Autodesk Fusion 360 part; units mm, degrees
sketch "Body" plane through (0, 0, 0) normal (0, 0, 1) x (1, 0, 0)
  circle A0 centre (0, 0) radius 85
  line L0 (-100, -41.4214) -> (-41.4214, -100)
  line L1 (-41.4214, -100) -> (41.4214, -100)
  line L2 (41.4214, -100) -> (100, -41.4214)
  line L3 (100, -41.4214) -> (100, 41.4214)
  line L4 (100, 41.4214) -> (41.4214, 100)
  line L5 (41.4214, 100) -> (-41.4214, 100)
  line L6 (-41.4214, 100) -> (-100, 41.4214)
  line L7 (-100, 41.4214) -> (-100, -41.4214)
  line L8 (-30.5, -100) -> (30.5, -100)
  line L9 (30.5, -100) -> (30.5, -120)
  line L10 (30.5, -120) -> (-30.5, -120)
  line L11 (-30.5, -120) -> (-30.5, -100)
  line L12 (-30.5, 100) -> (30.5, 100)
  line L13 (30.5, 100) -> (30.5, 120)
  line L14 (30.5, 120) -> (-30.5, 120)
  line L15 (-30.5, 120) -> (-30.5, 100)
  line L16 (100, 30.5) -> (120, 30.5)
  line L17 (120, 30.5) -> (120, -30.5)
  line L18 (120, -30.5) -> (100, -30.5)
  line L19 (100, -30.5) -> (100, 30.5)
  line L20 (-100, 30.5) -> (-120, 30.5)
  line L21 (-120, 30.5) -> (-120, -30.5)
  line L22 (-120, -30.5) -> (-100, -30.5)
  line L23 (-100, -30.5) -> (-100, 30.5)
  line L24 (-120, 0) -> (120, 0)
  line L25 (0, 120) -> (0, -120)
  dimension "d1" = 170
  dimension "d2" = 100
  dimension "d4" = 61
  dimension "d5" = 20
  dimension "d7" = 61
  dimension "d8" = 20
  dimension "d10" = 61
  dimension "d11" = 20
  dimension "d13" = 20
  dimension "d14" = 61
extrude "Extrude1" add sketch "Body" along normal blind 100 contours A0 L3 L4 L5 L12 L19 L24 L25 | L3 L16 L17 L19 L24 | L5 L12 L13 L14 L25
extrude "Extrude2" cut sketch "Body" along normal blind 7 contours L3 L16 L17 L19 L24 | L5 L12 L13 L14 L25
sketch "H_Circle" plane through (30.5, 0, 0) normal (1, 0, 0) x (0, 1, 0)
  line L0 (100, 7) -> (120, 7)
  line L1 (120, 7) -> (120, 100)
  line L2 (120, 100) -> (100, 100)
  line L3 (100, 100) -> (100, 7)
  line L4 (100, 100) -> (120, 100)
  line L5 (120, 100) -> (120, 7)
  line L6 (120, 7) -> (100, 7)
  line L7 (100, 7) -> (100, 100)
  line L8 (100, 100) -> (120, 100)
  line L9 (120, 100) -> (120, 80)
  line L10 (100, 80) -> (100, 100)
  line L11 (100, 7) -> (120, 7)
  line L12 (120, 7) -> (120, 27)
  line L13 (100, 27) -> (100, 7)
  circle A0 centre (110, 80) radius 6
  circle A1 centre (110, 80) radius 3
  circle A2 centre (110, 27) radius 6
  circle A3 centre (110, 27) radius 3
  dimension "d19" = 20
  dimension "d20" = 20
  dimension "d21" = 12
  dimension "d22" = 6
  dimension "d23" = 12
  dimension "d24" = 6
extrude "Extrude3" cut sketch "H_Circle" against normal blind 70 contours A1 | A3
extrude "Extrude4" cut sketch "H_Circle" against normal blind 6 contours A0 | A2
sketch "H_Hex" plane through (0, 30.5, 0) normal (0, 1, 0) x (-1, 0, 0)
  line L0 (-120, 7) -> (-100, 7)
  line L1 (-100, 7) -> (-100, 100)
  line L2 (-100, 100) -> (-120, 100)
  line L3 (-120, 100) -> (-120, 7)
  line L4 (-120, 100) -> (-100, 100)
  line L5 (-100, 100) -> (-100, 7)
  line L6 (-100, 7) -> (-120, 7)
  line L7 (-120, 7) -> (-120, 100)
  line L8 (-120, 100) -> (-100, 100)
  line L9 (-100, 100) -> (-100, 80)
  line L10 (-120, 80) -> (-120, 100)
  line L11 (-120, 7) -> (-100, 7)
  line L12 (-100, 7) -> (-100, 27)
  line L13 (-120, 27) -> (-120, 7)
  circle A0 centre (-110, 80) radius 3
  circle A1 centre (-110, 27) radius 3
  line L14 (-115.5, 76.8246) -> (-110, 73.6491)
  line L15 (-110, 73.6491) -> (-104.5, 76.8246)
  line L16 (-104.5, 76.8246) -> (-104.5, 83.1754)
  line L17 (-104.5, 83.1754) -> (-110, 86.3509)
  line L18 (-110, 86.3509) -> (-115.5, 83.1754)
  line L19 (-115.5, 83.1754) -> (-115.5, 76.8246)
  line L20 (-115.5, 23.8246) -> (-110, 20.6491)
  line L21 (-110, 20.6491) -> (-104.5, 23.8246)
  line L22 (-104.5, 23.8246) -> (-104.5, 30.1754)
  line L23 (-104.5, 30.1754) -> (-110, 33.3509)
  line L24 (-110, 33.3509) -> (-115.5, 30.1754)
  line L25 (-115.5, 30.1754) -> (-115.5, 23.8246)
  point P0 (-110, 80)
  point P1 (-110, 27)
  dimension "d30" = 20
  dimension "d31" = 20
  dimension "d32" = 6
  dimension "d33" = 6
  dimension "d34" = 5.5
  dimension "d35" = 5.5
extrude "Extrude5" cut sketch "H_Hex" against normal blind 5 contours L14 L15 L16 L17 L18 L19 | L20 L21 L22 L23 L24 L25
extrude "Extrude6" cut 2 faces at (110.2225, 30.5, 80.9749) (109.2094, 30.5, 26.0676) along direction (0, -1, 0) blind 80
Geometry check sheet. Reference: the model listing, model coordinates, mm. A direction names the side the tool comes from. Coordinates: 2 decimals unless noted, no trailing zeros. Order: outer loops, then holes, each group sorted by start corner. A loop starts at its lowest first (then second) coordinate and runs counter-clockwise, first axis right, second up. Notation, with made-up numbers: (29, 81.5) - (37, 81.5) arc R5 cw to (37, 87.5) - close; hole circle Ø3 at (55.25, 44.25). An arc over 180 degrees is marked (long way). Answer in a Markdown table with one row per item. Add a question column.
1. Section check C-C (z = 14). Enter the section's corners in (x, y), plus the area to 3 significant figures.
2. Section check B-B (y = 14.5). Enter the section's corners in (x, z).
3. Gauge pin test, flat ends, axial feed: pin 1 Ø10 at (x, y) = (10, 113) entering from -Z; pin 2 Ø6 at (x, z) = (25, 23) entering from -Y; pin 3 Ø3.5 at (y, z) = (107.5, 77.5) entering from +X; pin 4 Ø6 at (x, y) = (36.5, 71.5) entering from +Z. Record the tip position at first contact, or that the pin passes through.
4. Draft check along Y on faces 1 (the face through (27.54, 105.58, 84.06)), 2 (the face through (112.79, 28.04, 75.26)), 3 (the face through (59.4, 60.8, 49.3)). Enter one of: +Y half, -Y half, draft (parallel to the pull), parting line (faces both ways), or undercut.
5. Section check A-A (z = 80). Enter the section's corners in (x, y).
6. Material ranges on L1, parallel to Z at x = 29, y = 110; L2, parallel to Z at x = 110, y = 16; L3, parallel to Z at x = 8.5, y = 101.5, recorded low to high. Write a range as [from, to].
7. Section check D-D (x = 76.5). Enter the section's corners in (y, z).
8. Access from +Z, -Z, +X, -X, +Y, -Y to the whole of each face (thin tool, end or side, straight path). Record for faces 4 (the face through (15, 120, 53)), 5 (the face through (104.5, 28, 27)), 6 (the face through (24.5, 107, 79)).
Data:
| question | item | result |
|---|---|---|
| 1 | outline | (0, 85) arc R85 cw to (85, 0) - (120, 0) - (120, 30.5) - (100, 30.5) - (100, 41.42) - (41.42, 100) - (30.5, 100) - (30.5, 120) - (0, 120) - close |
| 1 | area | 3,830 mm² |
| 2 | outline | (83.75, 0) - (100, 0) - (100, 7) - (120, 7) - (120, 100) - (83.75, 100) - close; hole circle Ø6 at (110, 27); hole circle Ø6 at (110, 80) |
| 3 | pin 1 | stops at z = 7 |
| 3 | pin 2 | stops at y = 80.26 |
| 3 | pin 3 | stops at x = 24.5 |
| 3 | pin 4 | passes through |
| 4 | face 1 | undercut |
| 4 | face 2 | draft |
| 4 | face 3 | -Y half |
| 5 | outline | (0, 85) arc R85 cw to (85, 0) - (107, 0) - (107, 25.5) - (104.5, 25.5) - (104.5, 30.5) - (100, 30.5) - (100, 41.42) - (41.42, 100) - (30.5, 100) - (30.5, 104) - (24.5, 104) - (24.5, 107) - (0, 107) - close; (0, 113) - (24.5, 113) - (24.5, 116) - (30.5, 116) - (30.5, 120) - (0, 120) - close; (113, 0) - (120, 0) - (120, 30.5) - (115.5, 30.5) - (115.5, 25.5) - (113, 25.5) - close |
| 6 | L1 | z = [7, 21], [33, 74], [86, 100] |
| 6 | L2 | z = [7, 24], [30, 77], [83, 100] |
| 6 | L3 | z = [7, 100] |
| 7 | outline | (37.05, 0) - (64.92, 0) - (64.92, 100) - (37.05, 100) - close |
| 8 | face 4 | +Z, -Z, +X, -X, +Y |
| 8 | face 5 | +Y |
| 8 | face 6 | +X |
